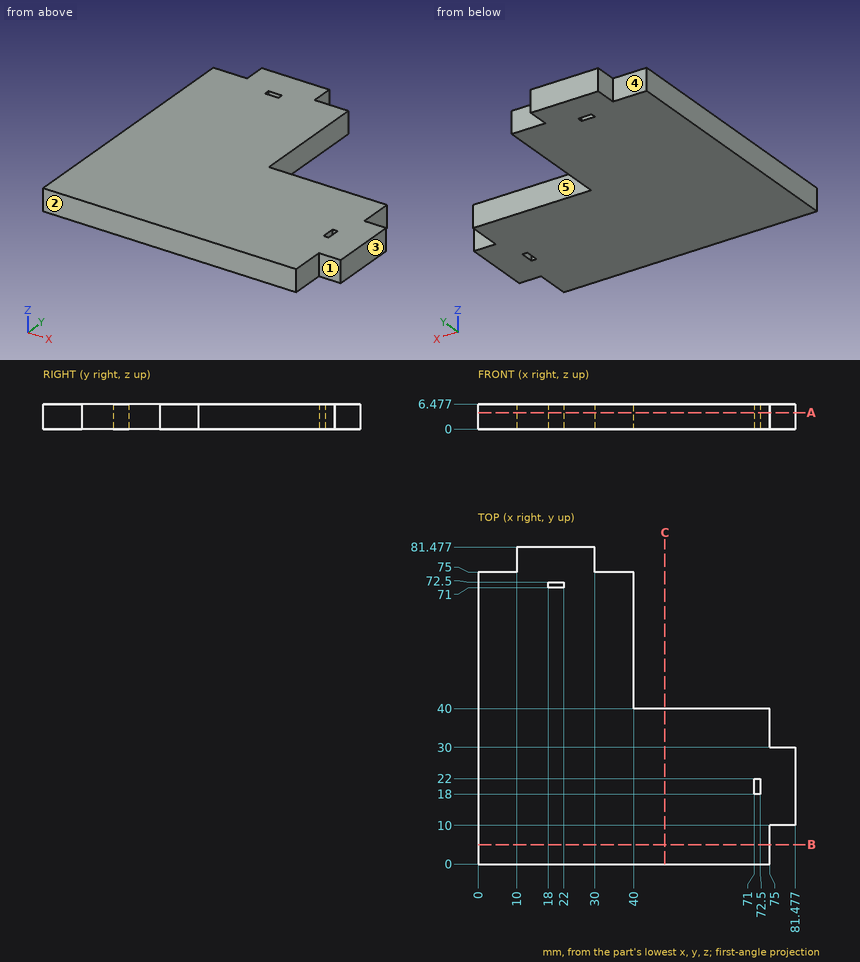
Input: dimensioned drawing with shaded views. Units: mm. Origin: part minimum x, y, z. A direction names the side the tool comes from. Coordinates: 2 decimals unless noted, no trailing zeros. Loops run counter-clockwise (first coordinate to the right, second up) from the corner with the lowest first, then second, coordinate; pieces in that order, holes last. Notation, with made-up numbers: M 32,61 L 89,61 A8 cw 89,75 Z; hole C -36,-9.5 d3. An arc over 180 degrees is marked long. Use a Markdown table: item, result. Add a question column.
1) Section B-B, the plane y = 5. Return the cut outline in (x, z), plus the area to 3 significant figures.
2) Pin query (flat end, axial travel): P1, Ø1.9, axis at x = 79, z = 4.5, coming from the -Y side; P2, Ø1.9, axis at x = 32.5, z = 2, coming from the +Y side; P3, Ø3, axis at y = 79, z = 2.5, coming from the -X side. Return the tip coordinate at first contact, or that it passes through.
3) Line query: L1, parallel to Y at x = 37, z = 5.5; L2, parallel to Y at x = 61.5, z = 1.25. Output: solid intervals per line, ascending. Write a range as from..to.
4) Section C-C, the plane x = 48. Return the cut outline in (y, z).
5) Set-up query: the marked faces 1, 2, 3, 4 and 5. Return all of +Z, -Z, +X, -X, +Y, -Y with unobstructed straight access to the full face (end or side cutting, diameter ignored); none if empty.
6) Section A-A, the plane z = 4.25. Return the cut outline in (x, y), plus the area to 3 significant figures.
Answer below:
| question | item | result |
|---|---|---|
| 1 | outline | M 0,0 L 75,0 L 75,6.48 L 0,6.48 Z |
| 1 | area | 486 mm2 |
| 2 | P1 | y = 10 |
| 2 | P2 | y = 75 |
| 2 | P3 | x = 10 |
| 3 | L1 | 0..75 |
| 3 | L2 | 0..40 |
| 4 | outline | M 0,0 L 40,0 L 40,6.48 L 0,6.48 Z |
| 5 | face 1 | +Z, -Z, +X, -Y |
| 5 | face 2 | +Z, -Z, +X, -X, -Y |
| 5 | face 3 | +Z, -Z, +X, +Y, -Y |
| 5 | face 4 | +Z, -Z, -X, +Y |
| 5 | face 5 | +Z, -Z, +X, +Y |
| 6 | outline | M 0,0 L 75,0 L 75,10 L 81.48,10 L 81.48,30 L 75,30 L 75,40 L 40,40 L 40,75 L 30,75 L 30,81.48 L 10,81.48 L 10,75 L 0,75 Z; hole M 18,71 L 22,71 L 22,72.5 L 18,72.5 Z; hole M 71,18 L 72.5,18 L 72.5,22 L 71,22 Z |
| 6 | area | 4,650 mm2 |
